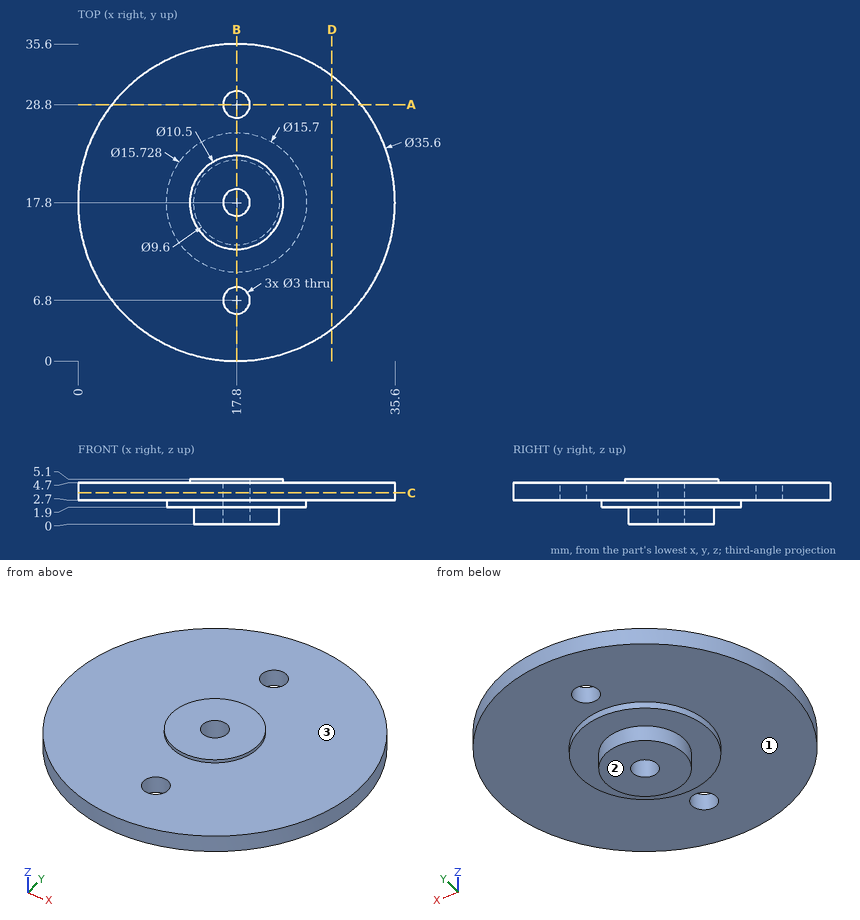
The figure shows three views and two pictorial views of one solid part (mm, origin at its lowest corner). Answer the questions. A direction names the side the tool comes from. Round coordinates to 2 decimals unless told otherwise and drop trailing zeros. Write each loop counter-clockwise with the first axis right and the second up, starting at its lowest first coordinate (ties: lowest second). Pieces come first, ordered by that corner, then holes. Notation, with made-up numbers: (-6, 55.5) - (15, 55.5) arc R15 cw to (15, 64.5) - close; hole circle Ø2 at (77, 76.25). An arc over 180 degrees is marked (long way). Answer in a Markdown table with one row per item. Add a question column.
1. A cutting plane is placed at D-D, the plane x = 28.5. Determine the outline of the cut face in (y, z) (3 decimals).
2. For the marked faces 1, 2 and 3, determine the directions among +Z, -Z, +X, -X, +Y, -Y from which every point of the face is accessible in a straight line to the end or side of a thin tool.
3. A cutting plane is placed at B-B, the plane x = 17.8. Count the separate pieces of the cut face and the enclosed holes in it, and give its area (3 significant figures).
4. A cutting plane is placed at A-A, the plane y = 28.8. Determine the outline of the cut face in (x, z).
5. Find the intervals of material crossed by line 1 along Y through (x, z) = (17.8, 3.8); line 2 along Z through (x, y) = (5, 9.5); line 3 along Z through (x, y) = (15.5, 24.5), in increasing order. Write a range as from..to.
6. A cutting plane is placed at C-C, the plane z = 3.55. Determine the outline of the cut face in (x, y), and give its area (3 significant figures).
7. Given pin 1 (2 mm diameter, centred on x = 14.5, z = 4.5, fed in from -Y); pin 2 (4 mm diameter, centred on x = 17.8, y = 28.8, fed in from +Z); pin 3 (1.5 mm diameter, centred on x = 6.5, y = 16.5, fed in from -Z), each flat-ended and moving along its own axis, determine where each tip first touches the part or whether it passes through.
Worked out:
| question | item | result |
|---|---|---|
| 1 | outline | (3.575, 2.7) - (32.025, 2.7) - (32.025, 4.7) - (3.575, 4.7) - close |
| 2 | face 1 | -Z |
| 2 | face 2 | -Z, +X, -X, +Y, -Y |
| 2 | face 3 | +Z |
| 3 | separate pieces | 4 |
| 3 | enclosed holes | 0 |
| 3 | area | 78.9 mm^2 |
| 4 | outline | (3.81, 2.7) - (16.3, 2.7) - (16.3, 4.7) - (3.81, 4.7) - close; (19.3, 2.7) - (31.79, 2.7) - (31.79, 4.7) - (19.3, 4.7) - close |
| 5 | line 1 | 0..5.3, 8.3..16.3, 19.3..27.3, 30.3..35.6 |
| 5 | line 2 | 2.7..4.7 |
| 5 | line 3 | 1.9..4.7 |
| 6 | outline | circle Ø35.6 at (17.8, 17.8); hole circle Ø3 at (17.8, 6.8); hole circle Ø3 at (17.8, 17.8); hole circle Ø3 at (17.8, 28.8) |
| 6 | area | 974 mm^2 |
| 7 | pin 1 | y = 0.15 |
| 7 | pin 2 | z = 4.7 |
| 7 | pin 3 | z = 2.7 |
